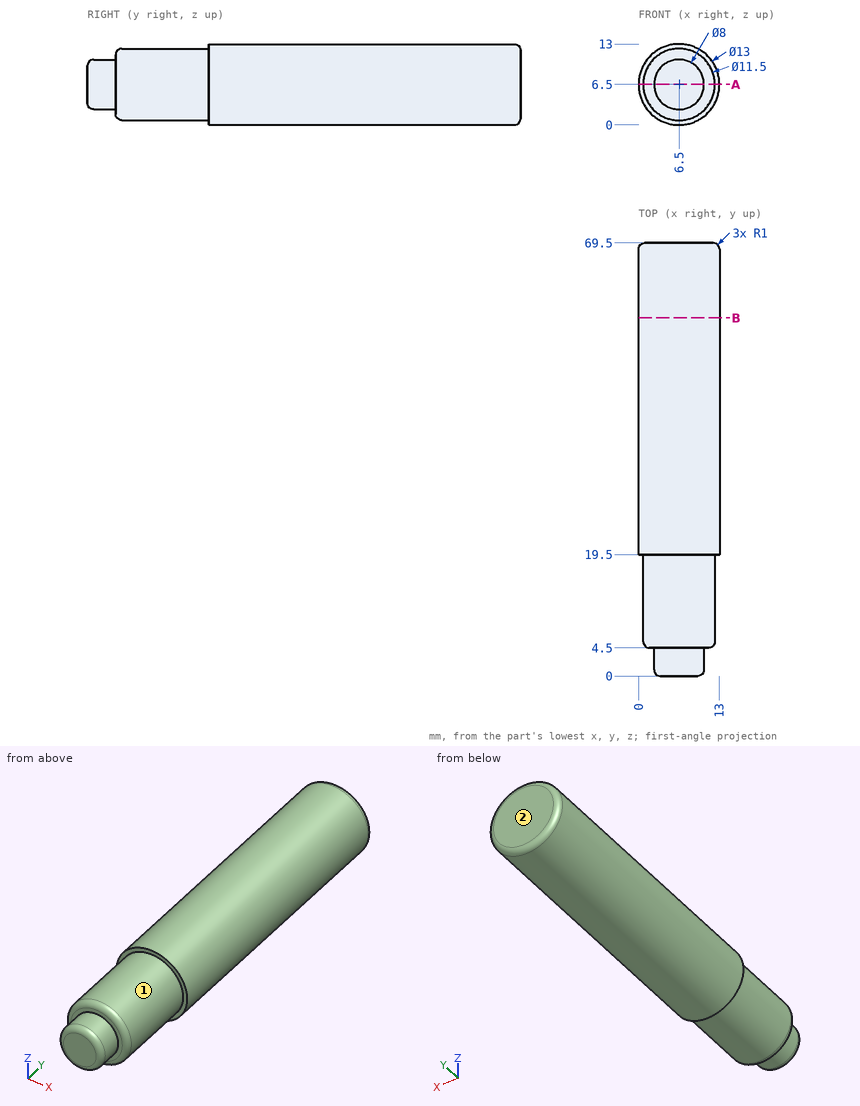
Drawing for the job (mm, zero at the part's lowest x, y, z). A direction names the side the tool comes from. Round coordinates to 2 decimals unless told otherwise and drop trailing zeros. Write each loop counter-clockwise with the first axis right and the second up, starting at its lowest first coordinate (ties: lowest second). Pieces come first, ordered by that corner, then holes.
Item 1: Band-saw the part on A-A on z = 6.5. Write the cut outline in (x, y).
Filled in:
outline: (0, 19.5) - (0.75, 19.5) - (0.75, 5.5) arc R1 ccw to (1.75, 4.5) - (2.5, 4.5) - (2.5, 1) arc R1 ccw to (3.5, 0) - (9.5, 0) arc R1 ccw to (10.5, 1) - (10.5, 4.5) - (11.25, 4.5) arc R1 ccw to (12.25, 5.5) - (12.25, 19.5) - (13, 19.5) - (13, 68.5) arc R1 ccw to (12, 69.5) - (1, 69.5) arc R1 ccw to (0, 68.5) - close
Item 2: Drill centre lines: L1, parallel to Y at x = 9, z = 10.5; L2, parallel to Z at x = 8, y = 6.5; L3, parallel to X at y = 20.5, z = 3.5. Where is each one in solid material? Low to high.
Filled in:
L1: y = 4.5 to 69.5
L2: z = 0.95 to 12.05
L3: x = 0.73 to 12.27
Item 3: Drop flat-ended pins along their axis: pin 1 Ø1.5 at (x, y) = (11, 52) entering from +Z; pin 2 Ø3 at (x, y) = (9.5, 46.5) entering from -Z. Give the stop position or say it passes through.
Filled in:
pin 1: stops at z = 11.81
pin 2: stops at z = 0.18
Item 4: Band-saw the part on B-B on y = 57.5. Write the cut outline in (x, z), then the cut area to 3 significant figures.
Filled in:
outline: circle Ø13 at (6.5, 6.5)
area: 133 mm2
Item 5: Tool access for the marked faces 1 and 2: list every direction of +Z, -Z, +X, -X, +Y, -Y with a clear straight run to the whole face (end or side of a thin tool).
Filled in:
face 1: -Y
face 2: +Z, -Z, +X, -X, +Y
